Verification items for the finished model (mm, model axes). A direction names the side the tool comes from. Coordinates: 2 decimals unless noted, no trailing zeros. Write each loop counter-clockwise with the first axis right and the second up, starting at its lowest first coordinate (ties: lowest second). Pieces come first, ordered by that corner, then holes. Notation, with made-up numbers: (42, 85.25) -> (83, 85.25) arc R27 cw to (83, 105.25) -> close; hole circle Ø6 at (77, 41). An arc over 180 degrees is marked (long way). Write item = value, one per line. Start each with the question number.
(1) Gauge pin test, flat ends, axial feed: pin 1 Ø8 at (x, y) = (-3.5, -10.5) entering from +Z; pin 2 Ø3 at (x, z) = (-20, 1) entering from -Y; pin 3 Ø3 at (y, z) = (1, 3) entering from -X; pin 4 Ø8 at (x, y) = (-4.5, 0) entering from +Z. Record the tip position at first contact, or that the pin passes through.
(2) Mould release check, pull along X, two halves, no side actions. Record for faces 3 (the face through (0, -12, 7)), 4 (the face through (0.625, -29.993, 3.451)): released by +X, released by -X, zero draft, split by the parting line, or undercut.
(3) Section check A-A (z = 5.25). Record the cut outline in (x, y).
(4) Material ranges on probe 1 along Y at (x, z) = (7, 2.25); probe 2 along X at (y, z) = (-15, 3.75); probe 3 along Y at (x, z) = (-11.5, 1.5), recorded low to high. Write a range as [from, to].
(5) Section check B-B (x = -23). State how many separate pieces and enclosed holes the cut face has, plus the area to 3 significant figures.
(6) Set-up check for faces 1 (the face through (23, 2.5, 3)), 2 (the face through (0, -12, 0)): record each of +Z, -Z, +X, -X, +Y, -Y from which the full face is reachable in a straight line by a thin tool's end or side.
```python
from build123d import *

# Parameters (mm, degrees)
F1_DEPTH = 7
F3_R     = 3.49999


# Not quite as in the source:
# - a fillet or chamfer that OpenCascade refuses, or shapes differently, is made with other operations: its cross-section is extruded or revolved along the edge and cut away or added
# - a fillet or chamfer is up to 0.001 mm smaller than in the source, because OpenCascade refuses the exact size


with BuildPart() as f1:
    # F0 (on Top) → F1 (new body)
    with BuildSketch(Plane.XY):
        with BuildLine():
            ThreePointArc((-29.8956518578, 2.5), (0, 30), (29.8956518578, 2.5))
            Line((29.8956518578, 2.5), (34.9106001094, 2.5))
            ThreePointArc((34.9106001094, 2.5), (0, 35), (-34.9106001094, 2.5))
            Line((-34.9106001094, 2.5), (-29.8956518578, 2.5))
        make_face()
        with BuildLine():
            Line((34.9106001094, 2.5), (29.8956518578, 2.5))
            ThreePointArc((29.8956518578, 2.5), (29.9739016123, 1.2510883797), (30, 0))
            ThreePointArc((30, 0), (29.9739016123, -1.2510883797), (29.8956518578, -2.5))
            Line((29.8956518578, -2.5), (34.9106001094, -2.5))
            ThreePointArc((34.9106001094, -2.5), (34.9776428868, -1.2507989787), (35, 0))
            ThreePointArc((35, 0), (34.9776428868, 1.2507989787), (34.9106001094, 2.5))
        make_face()
        with BuildLine():
            Line((34.9106001094, -2.5), (29.8956518578, -2.5))
            ThreePointArc((29.8956518578, -2.5), (0, -30), (-29.8956518578, -2.5))
            Line((-29.8956518578, -2.5), (-34.9106001094, -2.5))
            ThreePointArc((-34.9106001094, -2.5), (0, -35), (34.9106001094, -2.5))
        make_face()
        with BuildLine():
            ThreePointArc((-29.8956518578, -2.5), (-30, 0), (-29.8956518578, 2.5))
            Line((-29.8956518578, 2.5), (-34.9106001094, 2.5))
            ThreePointArc((-34.9106001094, 2.5), (-35, 0), (-34.9106001094, -2.5))
            Line((-34.9106001094, -2.5), (-29.8956518578, -2.5))
        make_face()
        with BuildLine():
            ThreePointArc((-16.1071412734, -2.5), (-16.3, 0), (-16.1071412734, 2.5))
            Line((-16.1071412734, 2.5), (-29.8956518578, 2.5))
            ThreePointArc((-29.8956518578, 2.5), (-30, 0), (-29.8956518578, -2.5))
            Line((-29.8956518578, -2.5), (-16.1071412734, -2.5))
        make_face()
        with BuildLine():
            ThreePointArc((-11.0199818512, -2.5), (-11.3, 0), (-11.0199818512, 2.5))
            Line((-11.0199818512, 2.5), (-16.1071412734, 2.5))
            ThreePointArc((-16.1071412734, 2.5), (-16.3, 0), (-16.1071412734, -2.5))
            Line((-16.1071412734, -2.5), (-11.0199818512, -2.5))
        make_face()
        with BuildLine():
            ThreePointArc((-11.0199818512, 2.5), (0, 11.3), (11.0199818512, 2.5))
            Line((11.0199818512, 2.5), (16.1071412734, 2.5))
            ThreePointArc((16.1071412734, 2.5), (0, 16.3), (-16.1071412734, 2.5))
            Line((-16.1071412734, 2.5), (-11.0199818512, 2.5))
        make_face()
        with BuildLine():
            Line((16.1071412734, -2.5), (11.0199818512, -2.5))
            ThreePointArc((11.0199818512, -2.5), (0, -11.3), (-11.0199818512, -2.5))
            Line((-11.0199818512, -2.5), (-16.1071412734, -2.5))
            ThreePointArc((-16.1071412734, -2.5), (0, -16.3), (16.1071412734, -2.5))
        make_face()
        with BuildLine():
            Line((29.8956518578, 2.5), (16.1071412734, 2.5))
            ThreePointArc((16.1071412734, 2.5), (16.2517137982, 1.2537139315), (16.3, 0))
            ThreePointArc((16.3, 0), (16.2517137982, -1.2537139315), (16.1071412734, -2.5))
            Line((16.1071412734, -2.5), (29.8956518578, -2.5))
            ThreePointArc((29.8956518578, -2.5), (29.9739016123, -1.2510883797), (30, 0))
            ThreePointArc((30, 0), (29.9739016123, 1.2510883797), (29.8956518578, 2.5))
        make_face()
        with BuildLine():
            ThreePointArc((11.0199818512, 2.5), (11.2297772667, 1.2578165768), (11.3, 0))
            ThreePointArc((11.3, 0), (11.2297772667, -1.2578165768), (11.0199818512, -2.5))
            Line((11.0199818512, -2.5), (16.1071412734, -2.5))
            ThreePointArc((16.1071412734, -2.5), (16.2517137982, -1.2537139315), (16.3, 0))
            ThreePointArc((16.3, 0), (16.2517137982, 1.2537139315), (16.1071412734, 2.5))
            Line((16.1071412734, 2.5), (11.0199818512, 2.5))
        make_face()
    extrude(amount=F1_DEPTH)

    # F2: fillet of radius 3.5 on 1 edges, made by hand

    # F2_s1 → F2_t2 (revolve, cut)
    with BuildSketch(Plane(origin=(0, 0, 0), x_dir=(0, 0, 1), z_dir=(0.0714285714, 0.9974457174, 0))):
        with BuildLine():
            ThreePointArc((3.5, -35), (5.9748737342, -33.9748737342), (7, -31.5))
            Line((7, -31.5), (7, -35))
            Line((7, -35), (3.5, -35))
        make_face()
    revolve(axis=Axis((0, 0, 7), (0, 0, 1)), mode=Mode.SUBTRACT)

    # F3 (radius 3.5 in the source; OpenCascade refuses exactly that, so slightly less here)
    f3_edges = [f1.edges().sort_by_distance(p)[0] for p in [
        (34.9106, -2.5, 0),
    ]]
    fillet(f3_edges, radius=F3_R)


solid = f1.part
```
Response:
q1.pin_1 = 7
q1.pin_2 = -29.07
q1.pin_3 = -35
q1.pin_4 = through
q2.face_3 = zero draft
q2.face_4 = undercut
q3.outline = circle Ø69.06 at (0, 0); hole (-29.9, -2.5) arc R30 ccw to (29.9, -2.5) -> (16.11, -2.5) arc R16.3 cw to (-16.11, -2.5) -> close; hole (-29.9, 2.5) -> (-16.11, 2.5) arc R16.3 cw to (16.11, 2.5) -> (29.9, 2.5) arc R30 ccw to start; hole circle Ø22.6 at (0, 0)
q4.probe_1 = [-34.06, -29.17], [-14.72, -8.87], [8.87, 14.72], [29.17, 34.06]
q4.probe_2 = [-31.61, -25.98], [-6.38, 6.38], [25.98, 31.61]
q4.probe_3 = [-32.39, -27.71], [-11.55, 11.55], [27.71, 32.39]
q5.separate_pieces = 3
q5.enclosed_holes = 0
q5.area = 120 mm2
q6.face_1 = +Z, -Z
q6.face_2 = -Z, +X, -X, +Y, -Y
